For this review, take the finished solid that the model builds, in its own axes (mm). Face numbers are marked on the shaded views. A direction names the side the tool comes from. Coordinates: 2 decimals unless noted, no trailing zeros. Loops run counter-clockwise (first coordinate to the right, second up) from the corner with the lowest first, then second, coordinate; pieces in that order, holes last. Notation, with made-up numbers: M 62,62.5 L 80,62.5 A27 ccw 80,95.5 Z; hole C -21.5,16.5 d1. An arc over 180 degrees is marked long. Answer as a JSON object with one key per item and string values. Group by question number.
Item 1: Mouldability with a two-part tool opening along X and no side actions: class the marked faces 3, 4 and 5 as +X half, -X half, draft (parallel to the pull), parting line (faces both ways), or undercut.
Item 2: Tool access review of the marked faces 1 and 2: name each direction out of +Z, -Z, +X, -X, +Y, -Y from which nothing blocks a thin tool from reaching the whole face with its end or side.
Item 3: Wall thickness on L1, parallel to Z at x = 0, y = -1.45; L2, parallel to Z at x = 0, y = 0.25: over which ranges is each line inside the solid? List them lowest first. Write a range as from..to.
Item 4: Add section B-B (x = 0). State the section outline as (y, z) points.
Item 5: Add section D-D (x = -3.75). State the section outline as (y, z) points, then the cut area to 3 significant figures.
Item 6: Add section A-A (z = 0). State the section outline as (x, y) points, then the cut area to 3 significant figures.
Item 7: Add section C-C (y = -0.45). State the section outline as (x, z) points, then the cut area to 3 significant figures.
Item 8: Insertion check: pin 1 (1 mm diameter, centred on y = 0.5, z = -2, fed in from +X). The pin has a flat end and moves straight along its axis. Give the tip position at first contact, or say it passes through.
from build123d import *

# Parameters (mm, degrees)
SKETCH_1_R          = 6
EXTRUDE_1_DEPTH     = 1
SKETCH_2_R          = 5
EXTRUDE_2_DEPTH     = 3
SKETCH_3_R          = 4
CUT_EXTRUDE_1_DEPTH = 2
SKETCH_4_R          = 2.25
CUT_EXTRUDE_2_DEPTH = 10


with BuildPart() as part:
    # 草图1 → 凸台-拉伸1 (new body)
    with BuildSketch(Plane(origin=(0, 0, 0), x_dir=(1, 0, 0), z_dir=(0, 1, 0))):
        Circle(SKETCH_1_R)
    extrude(amount=EXTRUDE_1_DEPTH)

    # 草图2 → 凸台-拉伸2 (add)
    with BuildSketch(Plane.XZ):
        Circle(SKETCH_2_R)
    extrude(amount=EXTRUDE_2_DEPTH)

    # 草图3 → 切除-拉伸1 (cut)
    with BuildSketch(Plane(origin=(0, 1, 0), x_dir=(1, 0, 0), z_dir=(0, 1, 0))):
        Circle(SKETCH_3_R)
    extrude(amount=-CUT_EXTRUDE_1_DEPTH, mode=Mode.SUBTRACT)

    # 草图4 → 切除-拉伸2 (cut)
    with BuildSketch(Plane(origin=(0, -1, 0), x_dir=(1, 0, 0), z_dir=(0, 1, 0))):
        Circle(SKETCH_4_R)
    extrude(amount=-CUT_EXTRUDE_2_DEPTH, mode=Mode.SUBTRACT)


solid = part.part
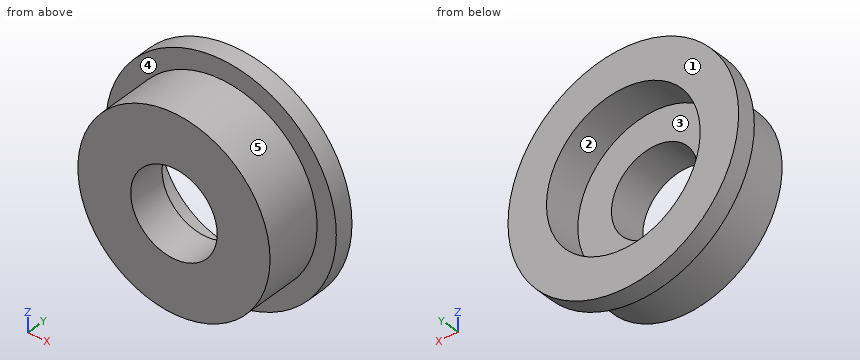
From the geometry:
{
 "1": {"face 3": "undercut", "face 4": "draft", "face 5": "parting line"},
 "2": {"face 1": "+Z, -Z, +X, -X, +Y", "face 2": "+Y"},
 "3": {"L1": "z = -5..-2.25, 2.25..5", "L2": "z = -6..-4, 4..6"},
 "4": {"outline": "M -3,-5 L 0,-5 L 0,-6 L 1,-6 L 1,-4 L -1,-4 L -1,-2.25 L -3,-2.25 Z; M -3,2.25 L -1,2.25 L -1,4 L 1,4 L 1,6 L 0,6 L 0,5 L -3,5 Z"},
 "5": {"outline": "M -3,-3.31 L 0,-3.31 L 0,-4.68 L 1,-4.68 L 1,-1.39 L -1,-1.39 L -1,1.39 L 1,1.39 L 1,4.68 L 0,4.68 L 0,3.31 L -3,3.31 Z", "area": "23.6 mm²"},
 "6": {"outline": "M -6,0 L -5,0 L -5,-3 L -2.25,-3 L -2.25,-1 L -4,-1 L -4,1 L -6,1 Z; M 2.25,-3 L 5,-3 L 5,0 L 6,0 L 6,1 L 4,1 L 4,-1 L 2.25,-1 Z", "area": "17.0 mm²"},
 "7": {"outline": "C 0,0 d10; hole C 0,0 d8", "area": "28.3 mm²"},
 "8": {"pin 1": "stops at x = 5.81"}
}
